Input: part model. Units: mm. Frame: model coordinates. A direction names the side the tool comes from. Coordinates: 2 decimals unless noted, no trailing zeros. Write each loop counter-clockwise with the first axis right and the second up, starting at its lowest first coordinate (ties: lowest second). Pieces come first, ordered by that corner, then holes. Notation, with made-up numbers: (-7.5, -33.75) -> (48.5, -33.75) arc R34 ccw to (48.5, 0.25) -> close; hole circle Ø4 at (41, 71). An arc over 180 degrees is marked (long way). Use one line per item in the form item = value. Start each with the question number.
(1) First-contact query: pin 1 (5 mm diameter, centred on y = 29, z = -3.5, fed in from +X); pin 2 (1.5 mm diameter, centred on y = -17, z = 2, fed in from +X); pin 3 (8 mm diameter, centred on y = -14.5, z = -6.5, fed in from -X). Flat tips, straight axial feed; report the tip coordinate or a pass-through.
(2) Cut plane A-A on x = 0. Return the cut outline in (y, z).
(3) Ray query, line 1 along Y through (x, z) = (7.5, 3.25); line 2 along Z through (x, y) = (-2, 13); line 3 along X through (y, z) = (22, -0.25). Return the intervals inside material, ascending.
(4) Set-up query: faces 4 (the face through (-4, 25, -3)), 5 (the face through (0, -12, -8.66)). Return all of +Z, -Z, +X, -X, +Y, -Y with unobstructed straight access to the full face (end or side cutting, diameter ignored); none if empty.
(5) Cut plane D-D on y = 32.5. Return the cut outline in (x, z).
(6) Pull-direction query (Y, two-part tool) for faces 1 (the face through (0, -25, 0)), 2 (the face through (-7.535, -12.325, -4.269)), 3 (the face through (0, 50, 0)); classes: released by +Y, released by -Y, zero draft, split by the parting line, or undercut.
(7) Cut plane C-C on z = 3.75. Return the cut outline in (x, y), plus the area to 3 significant figures.
(8) Cut plane B-B on y = -14. Return the cut outline in (x, z).
```python
from build123d import *

# Parameters (mm, degrees)
F1_DEPTH = 25
F2_DEPTH = 50


with BuildPart() as f1:
    # F0 (on Front) → F1 (new body)
    with BuildSketch(Plane.XZ):
        Polygon((-5, 0), (-5, 8.66), (-10.00044, 0), (-5, -8.66), align=None)
        with BuildLine():
            Line((5, -8.66), (5, 0))
            ThreePointArc((5, 0), (0, -5), (-5, 0))
            Line((-5, 0), (-5, -8.66))
            Line((-5, -8.66), (5, -8.66))
        make_face()
        with BuildLine():
            ThreePointArc((-5, 0), (0, -5), (5, 0))
            ThreePointArc((5, 0), (0, 5), (-5, 0))
        make_face()
        with BuildLine():
            Line((5, 0), (5, 8.66))
            Line((5, 8.66), (-5, 8.66))
            Line((-5, 8.66), (-5, 0))
            ThreePointArc((-5, 0), (0, 5), (5, 0))
        make_face()
        Polygon((10.00044, 0), (5, 8.66), (5, 0), (5, -8.66), align=None)
    extrude(amount=F1_DEPTH)

    # F0 (on Front) → F2 (join)
    with BuildSketch(Plane.XZ):
        with BuildLine():
            ThreePointArc((-5, 0), (0, -5), (5, 0))
            ThreePointArc((5, 0), (0, 5), (-5, 0))
        make_face()
    extrude(amount=-F2_DEPTH)


solid = f1.part
```
Values:
q1.pin_1 = 4.9
q1.pin_2 = 9.28
q1.pin_3 = -8.56
q2.outline = (-25, -8.66) -> (0, -8.66) -> (0, -5) -> (50, -5) -> (50, 5) -> (0, 5) -> (0, 8.66) -> (-25, 8.66) -> close
q3.line_1 = -25 to 0
q3.line_2 = -4.58 to 4.58
q3.line_3 = -4.99 to 4.99
q4.face_4 = +Y
q4.face_5 = -Z, +X, -X, +Y, -Y
q5.outline = circle Ø10 at (0, 0)
q6.face_1 = released by -Y
q6.face_2 = zero draft
q6.face_3 = released by +Y
q7.outline = (-7.84, -25) -> (7.84, -25) -> (7.84, 0) -> (3.31, 0) -> (3.31, 50) -> (-3.31, 50) -> (-3.31, 0) -> (-7.84, 0) -> close
q7.area = 722 mm2
q8.outline = (-10, 0) -> (-5, -8.66) -> (5, -8.66) -> (10, 0) -> (5, 8.66) -> (-5, 8.66) -> close
